Geometry check sheet. Reference: the model listing, model coordinates, mm. A direction names the side the tool comes from. Coordinates: 2 decimals unless noted, no trailing zeros. Loops run counter-clockwise (first coordinate to the right, second up) from the corner with the lowest first, then second, coordinate; pieces in that order, holes last. Notation, with made-up numbers: (-8.75, -16.75) -> (0.25, -16.75) arc R25 cw to (0.25, -1.75) -> close; hole circle Ø5 at (-8.75, 58.25). An arc over 180 degrees is marked (long way). Answer as a JSON object with one key per item and string values.
from build123d import *

# Parameters (mm, degrees)
SKETCH_1_R          = 2
EXTRUDE_1_DEPTH     = 12
SKETCH_6_R          = 16.5
EXTRUDE_3_DEPTH     = 10
SKETCH_7_R          = 2.5
CUT_EXTRUDE_3_DEPTH = 122.647030379
SKETCH_10_W         = 105
SKETCH_10_H         = 46
CUT_EXTRUDE_5_DEPTH = 6
FILLET_1_R          = 4


with BuildPart() as part:
    # 草图1 → 凸台-拉伸1 (new body)
    with BuildSketch(Plane.XY):
        with BuildLine():
            Line((10, -33), (-45, -33))
            Line((-45, -33), (-115, -33))
            Line((-115, -33), (-115, 33))
            Line((-115, 33), (-45, 33))
            Line((-45, 33), (10, 33))
            Line((10, 33), (45, 21.5))
            ThreePointArc((45, 21.5), (66.5, 0), (45, -21.5))
            Line((45, -21.5), (10, -33))
        make_face()
        with Locations((-35, 10)):
            Circle(SKETCH_1_R, mode=Mode.SUBTRACT)
        with Locations((-25, 10)):
            Circle(SKETCH_1_R, mode=Mode.SUBTRACT)
        with Locations((-25, -10)):
            Circle(SKETCH_1_R, mode=Mode.SUBTRACT)
        with Locations((-35, -10)):
            Circle(SKETCH_1_R, mode=Mode.SUBTRACT)
        with Locations((-55, 10)):
            Circle(SKETCH_1_R, mode=Mode.SUBTRACT)
        with Locations((-55, -10)):
            Circle(SKETCH_1_R, mode=Mode.SUBTRACT)
        with Locations((-45, -10)):
            Circle(SKETCH_1_R, mode=Mode.SUBTRACT)
        with Locations((-45, 10)):
            Circle(SKETCH_1_R, mode=Mode.SUBTRACT)
        with Locations((-75, 10)):
            Circle(SKETCH_1_R, mode=Mode.SUBTRACT)
        with Locations((-75, -10)):
            Circle(SKETCH_1_R, mode=Mode.SUBTRACT)
        with Locations((-65, -10)):
            Circle(SKETCH_1_R, mode=Mode.SUBTRACT)
        with Locations((-65, 10)):
            Circle(SKETCH_1_R, mode=Mode.SUBTRACT)
        with Locations((-95, 10)):
            Circle(SKETCH_1_R, mode=Mode.SUBTRACT)
        with Locations((-95, -10)):
            Circle(SKETCH_1_R, mode=Mode.SUBTRACT)
        with Locations((-85, -10)):
            Circle(SKETCH_1_R, mode=Mode.SUBTRACT)
        with Locations((-85, 10)):
            Circle(SKETCH_1_R, mode=Mode.SUBTRACT)
    extrude(amount=EXTRUDE_1_DEPTH)

    # 草图6 → 凸台-拉伸3 (add)
    with BuildSketch(Plane(origin=(0, 0, 0), x_dir=(-1, 0, 0), z_dir=(0, 0, -1))):
        with Locations((-45, 0)):
            Circle(SKETCH_6_R)
    extrude(amount=EXTRUDE_3_DEPTH)

    # 草图7 → 切除-拉伸3 (cut, through all)
    with BuildSketch(Plane(origin=(0, 0, -10), x_dir=(-1, 0, 0), z_dir=(0, 0, -1))):
        with Locations((-51, 10.392304845)):
            Circle(SKETCH_7_R)
        with Locations((-39, 10.392304845)):
            Circle(SKETCH_7_R)
        with Locations((-33, 0)):
            Circle(SKETCH_7_R)
        with Locations((-39, -10.392304845)):
            Circle(SKETCH_7_R)
        with Locations((-51, -10.392304845)):
            Circle(SKETCH_7_R)
        with Locations((-57, 0)):
            Circle(SKETCH_7_R)
    extrude(amount=-CUT_EXTRUDE_3_DEPTH, mode=Mode.SUBTRACT)

    # 草图10 → 切除-拉伸5 (cut)
    with BuildSketch(Plane.XY.offset(12)):
        with Locations((-62.5, 0)):
            Rectangle(SKETCH_10_W, SKETCH_10_H)
    extrude(amount=-CUT_EXTRUDE_5_DEPTH, mode=Mode.SUBTRACT)

    # 圆角1
    fillet_1_edges = [part.edges().sort_by_distance(p)[0] for p in [
        (-52.5, 33, 0),
        (-52.5, -33, 0),
        (-115, 0, 0),
    ]]
    fillet(fillet_1_edges, radius=FILLET_1_R)


solid = part.part
1. Mould release check, pull along X, two halves, no side actions. Record for faces 3 (the face through (27.74, -27.17, 5.92)), 4 (the face through (-63, -23, 9)), 5 (the face through (-56.474, -8.648, 2.958)): released by +X, released by -X, zero draft, split by the parting line, or undercut.
Evaluation:
{"face 3": "released by +X", "face 4": "zero draft", "face 5": "undercut"}
2. Section check C-C, the plane x = 57. Record the boundary of the cut face in (y, z), then the cut area to 3 significant figures.
Evaluation:
{"outline": "(-17.84, 0) -> (-11.32, 0) -> (-11.32, -10) -> (-2.5, -10) -> (-2.5, 12) -> (-17.84, 12) -> close; (2.5, -10) -> (11.32, -10) -> (11.32, 0) -> (17.84, 0) -> (17.84, 12) -> (2.5, 12) -> close", "area": "545 mm^2"}
3. Depth check by flat-ended pin: P1, Ø4.5, axis at x = -85, y = 10, coming from the +Z side; P2, Ø12, axis at x = -38, z = -4.5, coming from the +Y side; P3, Ø5, axis at x = 6, y = -0.5, coming from the -Z side. Enter the tip coordinate at first touch or a pass-through.
Evaluation:
{"P1": "stops at z = 6", "P2": "stops at y = 32.12", "P3": "stops at z = 0"}
4. Tool access check on faces 1 (the face through (-63, 23, 9)), 2 (the face through (35.5, 0.1, 0.8)). Record the directions out of +Z, -Z, +X, -X, +Y, -Y that give a thin tool (end or side, any length) a straight path to the whole face; none if there is none.
Evaluation:
{"face 1": "+Z, -X", "face 2": "+Z, -Z"}
5. Section check D-D, the plane y = 4.5. Record the boundary of the cut face in (x, z).
Evaluation:
{"outline": "(-115, 4) arc R4 ccw to (-111, 0) -> (29.13, 0) -> (29.13, -10) -> (60.87, -10) -> (60.87, 0) -> (66.02, 0) -> (66.02, 12) -> (-10, 12) -> (-10, 6) -> (-115, 6) -> close"}
6. Thickness scan on probe 1 along Y at (x, z) = (-65, 4.4); probe 2 along Y at (x, z) = (39, 6); probe 3 along Y at (x, z) = (-61, 8). Record the ranges inside material, lowest first. Write a range as from..to.
Evaluation:
{"probe 1": "y = -33..-12, -8..8, 12..33", "probe 2": "y = -23.47..-12.89, -7.89..7.89, 12.89..23.47", "probe 3": "y = -33..-23, 23..33"}
7. Section check B-B, the plane z = 8.5. Record the boundary of the cut face in (x, y), then the cut area to 3 significant figures.
Evaluation:
{"outline": "(-115, -33) -> (10, -33) -> (45, -21.5) arc R21.5 ccw to (45, 21.5) -> (10, 33) -> (-115, 33) -> (-115, 23) -> (-10, 23) -> (-10, -23) -> (-115, -23) -> close; hole circle Ø5 at (33, 0); hole circle Ø5 at (39, -10.39); hole circle Ø5 at (39, 10.39); hole circle Ø5 at (51, -10.39); hole circle Ø5 at (51, 10.39); hole circle Ø5 at (57, 0)", "area": "5,940 mm^2"}
8. Section check A-A, the plane x = -25. Record the boundary of the cut face in (y, z).
Evaluation:
{"outline": "(-33, 4) arc R4 ccw to (-29, 0) -> (-12, 0) -> (-12, 6) -> (-23, 6) -> (-23, 12) -> (-33, 12) -> close; (-8, 0) -> (8, 0) -> (8, 6) -> (-8, 6) -> close; (12, 0) -> (29, 0) arc R4 ccw to (33, 4) -> (33, 12) -> (23, 12) -> (23, 6) -> (12, 6) -> close"}
